Model file for the job. Use its own axes, mm. Face numbers are marked on the shaded views. A direction names the side the tool comes from. Give positions to 0.01 mm unless a question says otherwise; leave off trailing zeros. Write each loop counter-clockwise with the first axis right and the second up, starting at its lowest first coordinate (ties: lowest second). Pieces come first, ordered by that corner, then holes. Notation, with made-up numbers: (79, 1) - (99, 1) arc R18 ccw to (99, 22) - close; hole circle Ø8 at (22, 26.25). An arc over 180 degrees is marked (long way). One line per item, written item: value. Start each with the question number.
(1) Cut at A-A, the plane y = -34.35. List the corners of the cut face in (x, z), and give its area (3 significant figures).
(2) Cut at B-B, the plane z = 5.5. List the corners of the cut face in (x, y), and give its area (3 significant figures).
(3) Probe L1, parallel to X at y = -36.75, z = 7.75; L2, parallel to X at y = -34.1, z = 13.5; L3, parallel to Z at x = -6.75, y = -35.75. List the from-to ranges inside material, lowest first.
(4) 3-axis set-ups, long thin cutter, end or side, ignore diameter. For the marked faces 1, 2 and 3: which of +Z, -Z, +X, -X, +Y, -Y reach the whole face in a straight line?
(5) Drop flat-ended pins along their axis: P1, Ø2, axis at x = 13, y = -35.5, coming from the +Z side; P2, Ø2, axis at x = 13, y = -34.5, coming from the -Z side; P3, Ø1.5, axis at x = -8.5, y = -35.5, coming from the +Z side. Give the stop position or say it passes through.
(6) Cut at C-C, the plane x = -8. List the corners of the cut face in (y, z).
from build123d import *

# Parameters (mm, degrees)
SKETCH009_W  = 24
SKETCH009_H  = 13
PAD005_DEPTH = 4
FILLET001_R  = 6
SKETCH010_W  = 5.5
SKETCH010_H  = 5.5
PAD006_DEPTH = 4


with BuildPart() as part:
    # Sketch009 (on DatumPlane) → Pad005 (new body)
    with BuildSketch(Plane.XZ.offset(33)):
        with Locations((0, 8.5)):
            Rectangle(SKETCH009_W, SKETCH009_H)
    extrude(amount=PAD005_DEPTH)

    # Fillet001
    fillet001_edges = [part.edges().sort_by_distance(p)[0] for p in [
        (-12, -35, 15),
        (12, -35, 15),
        (-12, -35, 2),
        (12, -35, 2),
    ]]
    fillet(fillet001_edges, radius=FILLET001_R)

    # Sketch010 (on DatumPlane) → Pad006 (join)
    with BuildSketch(Plane.XZ.offset(33)):
        with Locations((12.75, 8.5)):
            Rectangle(SKETCH010_W, SKETCH010_H)
    extrude(amount=PAD006_DEPTH)


solid = part.part
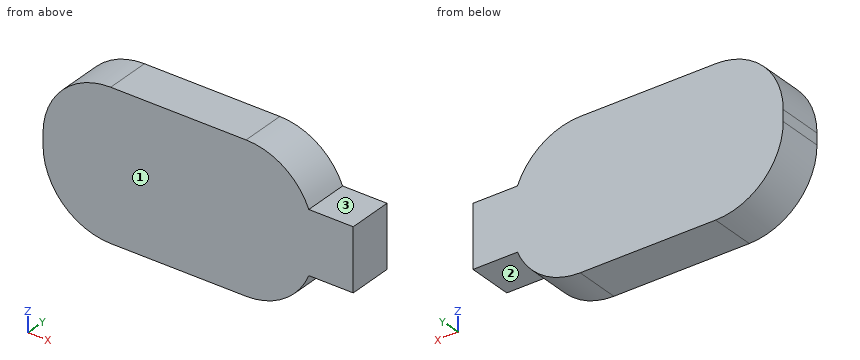
Answers follow:
1. outline: (-12, 8) arc R6 ccw to (-6, 2) - (6, 2) arc R6 ccw to (11.56, 5.75) - (15.5, 5.75) - (15.5, 11.25) - (11.56, 11.25) arc R6 ccw to (6, 15) - (-6, 15) arc R6 ccw to (-12, 9) - close
1. area: 301 mm²
2. outline: (-11.45, -37) - (11.45, -37) - (11.45, -33) - (-11.45, -33) - close
2. area: 91.6 mm²
3. L1: x = -11.99 to 15.5
3. L2: x = -9.97 to 9.97
3. L3: z = 2.05 to 14.95
4. face 1: +Z, -Z, +X, -X, -Y
4. face 2: -Z, +X, +Y, -Y
4. face 3: +Z, +X, +Y, -Y
5. P1: stops at z = 11.25
5. P2: stops at z = 5.75
5. P3: stops at z = 14.74
6. outline: (-37, 2.34) - (-33, 2.34) - (-33, 14.66) - (-37, 14.66) - close
